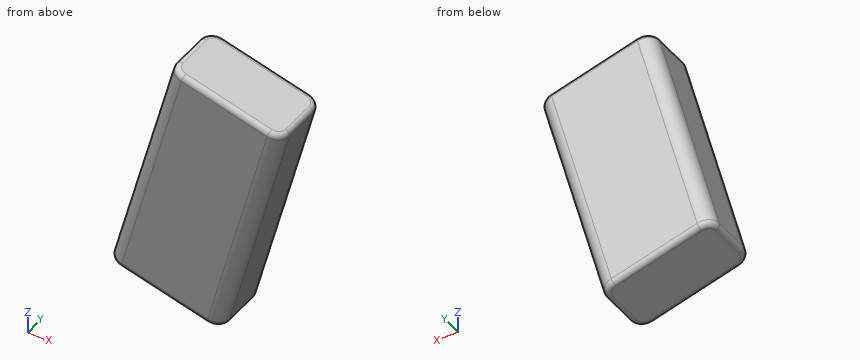
```python
from build123d import *

# Parameters (mm, degrees)
SKETCH_W             = 33.5
SKETCH_H             = 69
PAD_DEPTH            = 9.25
FILLET_R             = 4
FILLET001_R          = 1.5
BODY_PLACEMENT_ANGLE = 15


with BuildPart() as part:
    # Sketch → Pad (new body, symmetric)
    with BuildSketch(Plane.XZ):
        Rectangle(SKETCH_W, SKETCH_H)
    extrude(amount=PAD_DEPTH, both=True)

    # Fillet
    fillet_edges = [part.edges().sort_by_distance(p)[0] for p in [
        (-16.75, -9.25, 0),
        (-16.75, 9.25, 0),
        (16.75, -9.25, 0),
        (16.75, 9.25, 0),
    ]]
    fillet(fillet_edges, radius=FILLET_R)

    # Fillet001
    fillet001_edges = [part.edges().sort_by_distance(p)[0] for p in [
        (-16.75, 0, 34.5),
        (-15.578427, 8.078427, 34.5),
        (-15.578427, -8.078427, 34.5),
        (0, 9.25, 34.5),
        (0, -9.25, 34.5),
        (15.578427, 8.078427, 34.5),
        (15.578427, -8.078427, 34.5),
        (16.75, 0, 34.5),
        (16.75, 0, -34.5),
        (15.578427, 8.078427, -34.5),
        (15.578427, -8.078427, -34.5),
        (0, 9.25, -34.5),
        (0, -9.25, -34.5),
        (-15.578427, 8.078427, -34.5),
        (-15.578427, -8.078427, -34.5),
        (-16.75, 0, -34.5),
    ]]
    fillet(fillet001_edges, radius=FILLET001_R)


with BuildPart() as part_1:
    # Body placement: moved
    add(part.part.moved(Location((-42.5512320173, 0, -60.1655412245))).rotate(Axis((-42.5512320173, 0, -60.1655412245), (0, 1, 0)), BODY_PLACEMENT_ANGLE))


solid = part_1.part
```
The model under review builds one solid part; all positions refer to its coordinate system, in mm. Coordinates: 2 decimals unless noted, no trailing zeros. Order: outer loops, then holes, each group sorted by start corner. A loop starts at its lowest first (then second) coordinate and runs counter-clockwise, first axis right, second up. Notation, with made-up numbers: (-35.5, 76.25) -> (-23.5, 76.25) arc R32 cw to (-23.5, 110.25) -> close; hole circle Ø11 at (11.25, 17). An arc over 180 degrees is marked (long way). Answer in a Markdown table with one row per item. Add a question column.
Item 1: Clearance check with flat-ended pins moving along their axes: pin 1 (5 mm diameter, centred on y = -3.5, z = -52.5, fed in from -X); pin 2 (8 mm diameter, centred on y = -7, z = -61, fed in from +X); pin 3 (10 mm diameter, centred on y = -4.5, z = -72, fed in from +X). State where each tip first meets the part, or that it passes through.
Item 2: To check wall thickness, follow probe 1 along X at (y, z) = (6.75, -66); probe 2 along X at (y, z) = (4.5, -76.5); probe 3 along Z at (x, y) = (-47, -2.75). State the ranges of each line that lie inside material, in increasing order.
Item 3: We need section A-A on y = 2. Write out the cut boundary in (x, z), plus the area to 3 significant figures.
Final values:
| question | item | result |
|---|---|---|
| 1 | pin 1 | stops at x = -58.51 |
| 1 | pin 2 | stops at x = -24.45 |
| 1 | pin 3 | stops at x = -27.04 |
| 2 | probe 1 | x = -61.15 to -27.08 |
| 2 | probe 2 | x = -64.27 to -29.59 |
| 2 | probe 3 | z = -94.69 to -23.26 |
| 3 | outline | (-67.27, -87.71) arc R1.5 ccw to (-66.21, -89.54) -> (-36.75, -97.44) arc R1.5 ccw to (-34.91, -96.38) -> (-17.83, -32.63) arc R1.5 ccw to (-18.89, -30.79) -> (-48.35, -22.89) arc R1.5 ccw to (-50.19, -23.95) -> close |
| 3 | area | 2,310 mm2 |
